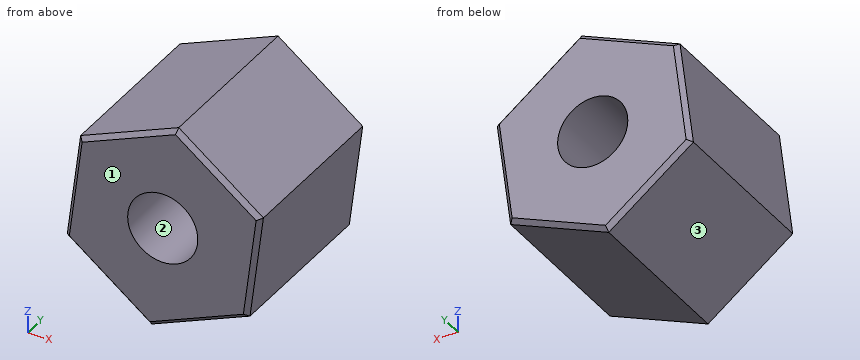
Autodesk Inventor part; units mm, degrees
ref_plane "YZ Plane" through (0, 0, 0) normal (1, 0, 0) x (0, 1, 0)
ref_plane "XZ Plane" through (0, 0, 0) normal (0, 1, 0) x (-1, 0, 0)
ref_plane "XY Plane" through (0, 0, 0) normal (0, 0, 1) x (1, 0, 0)
sketch "Sketch1" plane through (0, 0, 0) normal (0, 1, 0) x (-1, 0, 0)
  circle A0 centre (0, 0) radius 4
  line L0 (11.1804, -4.6903) -> (1.5283, -12.0276)
  line L1 (1.5283, -12.0276) -> (-9.6521, -7.3374)
  line L2 (-9.6521, -7.3374) -> (-11.1804, 4.6903)
  line L3 (-11.1804, 4.6903) -> (-1.5283, 12.0276)
  line L4 (-1.5283, 12.0276) -> (9.6521, 7.3374)
  line L5 (9.6521, 7.3374) -> (11.1804, -4.6903)
  dimension "d0" = 8
  dimension "d19" = 10.5
extrude "Extrusion1" add sketch "Sketch1" along normal blind 20
thread "Thread1"
chamfer "Chamfer1" distance 0.5 angle 45 12 edges at (-4.0619, 0, 9.6825) (6.3543, 0, 8.359) (10.4162, 0, -1.3235) (4.0619, 0, -9.6825) (-6.3543, 0, -8.359) (-10.4162, 0, 1.3235) (-4.0619, 20, 9.6825) (-10.4162, 20, 1.3235) (6.3543, 20, 8.359) (-6.3543, 20, -8.359) (4.0619, 20, -9.6825) (10.4162, 20, -1.3235)
properties part number "5M nut 20mm" material "Iron, Gray"
Build history of the part. All positions in model axes, mm. Face numbers are marked on the shaded views. Coordinates: 2 decimals unless noted, no trailing zeros. Order: outer loops, then holes, each group sorted by start corner. A loop starts at its lowest first (then second) coordinate and runs counter-clockwise, first axis right, second up. Notation, with made-up numbers: (-36.5, 7.5) -> (-26.5, 7.5) arc R16 cw to (-26.5, 32.5) -> close; hole circle Ø3 at (-36.5, 49.5). An arc over 180 degrees is marked (long way). Answer in a Markdown table with one row per item. Add a question column.
Q1. Band-saw the part on B-B, the plane x = 0. List the corners of the cut face in (y, z).
Q2. Band-saw the part on A-A, the plane y = 16. List the corners of the cut face in (x, z).
Q3. Drop flat-ended pins along their axis: pin 1 (2 mm diameter, centred on y = 8.5, z = -4.5, fed in from +X); pin 2 (1 mm diameter, centred on x = 0.5, y = 12.5, fed in from +Z); pin 3 (1.5 mm diameter, centred on y = 10.5, z = 2.5, fed in from +X). Give the stop position or say it passes through.
Q4. Wall check: line 1 along Z through (x, y) = (0, 5.25); line 2 along Y through (x, z) = (-6.5, -8); line 3 along X through (y, z) = (10.25, -3). Give the ranges that are in metal, low to high. Write a range as [from, to].
Q5. Band-saw the part on C-C, the plane z = 0. List the corners of the cut face in (x, y), then the cut area to 3 significant figures.
Q6. Band-saw the part on D-D, the plane x = -6.75. List the corners of the cut face in (y, z), then the cut area to 3 significant figures.
Q7. Mould opens along Z. For the marked faces 1, 2 and 3 say: +Z half, -Z half, draft (parallel to the pull), parting line (faces both ways), or undercut.
Answers follow:
| question | item | result |
|---|---|---|
| 1 | outline | (0, -10.84) -> (0.5, -11.39) -> (19.5, -11.39) -> (20, -10.84) -> (20, -4) -> (0, -4) -> close; (0, 4) -> (20, 4) -> (20, 10.84) -> (19.5, 11.39) -> (0.5, 11.39) -> (0, 10.84) -> close |
| 2 | outline | (-11.18, -4.69) -> (-1.53, -12.03) -> (9.65, -7.34) -> (11.18, 4.69) -> (1.53, 12.03) -> (-9.65, 7.34) -> close; hole circle Ø8 at (0, 0) |
| 3 | pin 1 | x = 10.14 |
| 3 | pin 2 | z = 11.81 |
| 3 | pin 3 | x = 11 |
| 4 | line 1 | [-11.39, -4], [4, 11.39] |
| 4 | line 2 | [0.3, 19.7] |
| 4 | line 3 | [-10.97, -2.65], [2.65, 10.2] |
| 5 | outline | (-10.58, 0.5) -> (-10.08, 0) -> (-4, 0) -> (-4, 20) -> (-10.08, 20) -> (-10.58, 19.5) -> close; (4, 0) -> (10.08, 0) -> (10.58, 0.5) -> (10.58, 19.5) -> (10.08, 20) -> (4, 20) -> close |
| 5 | area | 263 mm^2 |
| 6 | outline | (0, -7.43) -> (0.5, -8.06) -> (19.5, -8.06) -> (20, -7.43) -> (20, 8.01) -> (19.5, 8.55) -> (0.5, 8.55) -> (0, 8.01) -> close |
| 6 | area | 332 mm^2 |
| 7 | face 1 | draft |
| 7 | face 2 | undercut |
| 7 | face 3 | -Z half |
